from build123d import *

# Parameters (mm, degrees)
F1_DEPTH = 69.342
F4_DEPTH = 107.442
F6_DEPTH = 136.652
F7_R     = 6.789737
F7_R_2   = 6.259827
F8_DEPTH = 85.344


with BuildPart() as f1:
    # F0 (on Front) → F1 (new body)
    with BuildSketch(Plane.XZ):
        Polygon((0, 38.1), (-38.1, 38.1), (-38.1, 0), (0, 0), (38.1, 0), (38.1, 38.1), align=None)
    extrude(amount=F1_DEPTH)

    # F3 (on offset) → F4 (join)
    with BuildSketch(Plane.XZ.offset(78.994)):
        with BuildLine():
            Line((16.352327, 39.380998), (-16.352311, 39.378844))
            ThreePointArc((-16.352311, 39.378844), (0.001077, 23.146536), (16.352327, 39.380998))
        make_face()
    extrude(amount=-F4_DEPTH)

    # F5 (on offset) → F6 (cut)
    with BuildSketch(Plane.XZ.offset(78.994)):
        with BuildLine():
            Line((0, 39.475866), (-7.966925, 39.475866))
            ThreePointArc((-7.966925, 39.475866), (-0.026347, 31.508984), (7.966751, 39.423171))
            Line((7.966751, 39.423171), (0, 39.475866))
        make_face()
    extrude(amount=-F6_DEPTH, mode=Mode.SUBTRACT)

    # F7 (on Top) → F8 (cut)
    with BuildSketch(Plane.XY):
        with Locations((-27.498437, -37.382606)):
            Circle(F7_R)
        with Locations((27.498439, -37.382606)):
            Circle(F7_R_2)
    extrude(amount=F8_DEPTH, mode=Mode.SUBTRACT)


solid = f1.part
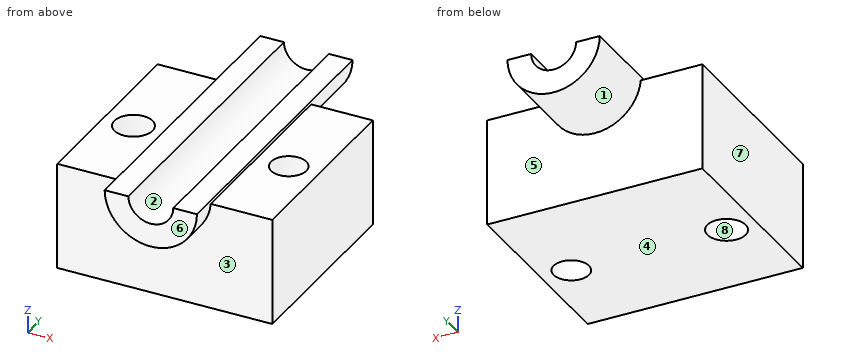
Input: part model. Units: mm. Frame: model coordinates. Face numbers are marked on the shaded views. A direction names the side the tool comes from. Coordinates: 2 decimals unless noted, no trailing zeros. Order: outer loops, then holes, each group sorted by start corner. A loop starts at its lowest first (then second) coordinate and runs counter-clockwise, first axis right, second up. Notation, with made-up numbers: M 38.25,37 L 57.25,37 A16 ccw 57.25,57 Z; hole C 59,-25.75 d2. An arc over 180 degrees is marked long. Answer in a Markdown table with one row per item.
(1) Contact query for flat-ended pins moving along their axis: pin 1 Ø19 at (x, z) = (-4.5, 14.5) entering from +Y; pin 2 Ø17.5 at (x, y) = (-25.5, -25) entering from +Z; pin 3 Ø1.5 at (x, z) = (27, 30) entering from -Y; pin 4 Ø2 at (x, z) = (-22, 19) entering from +Y. Output: stop coordinate, or through.
Numbers:
| item | result |
|---|---|
| pin 1 | stops at y = 28.45 |
| pin 2 | stops at z = 38.1 |
| pin 3 | stops at y = -69.34 |
| pin 4 | stops at y = 0 |
(2) Draft query along Y for the marked faces 6, 7 and 8. Return one class per face: pulls with the +Y half, pulls with the -Y half, needs draft (parallel to the pull), parting line crosses it, or undercut.
Numbers:
| item | result |
|---|---|
| face 6 | pulls with the -Y half |
| face 7 | needs draft |
| face 8 | undercut |
(3) Access query for the marked faces 1, 2, 3, 4 and 5. Directions: +Z, -Z, +X, -X, +Y, -Y. A direction counts if a zero-diameter tool reaches every point of the face in a straight line with its end or side. Return the directions, or none.
Numbers:
| item | result |
|---|---|
| face 1 | none |
| face 2 | +Z, +Y, -Y |
| face 3 | -Z, -Y |
| face 4 | -Z, +X, -X, +Y, -Y |
| face 5 | -Z, +Y |
(4) Section query C-C, the plane x = 0. Output: boundary loops of the cut face in (y, z), plus the area to 3 significant figures.
Numbers:
| item | result |
|---|---|
| outline | M -78.99,23.15 L -69.34,23.15 L -69.34,0 L 0,0 L 0,23.15 L 28.45,23.15 L 28.45,31.51 L -78.99,31.51 Z |
| area | 2,500 mm^2 |
(5) Section query A-A, the plane x = -31. Output: boundary loops of the cut face in (y, z), plus the area to 3 significant figures.
Numbers:
| item | result |
|---|---|
| outline | M -69.34,0 L -43.2,0 L -43.2,38.1 L -69.34,38.1 Z; M -31.57,0 L 0,0 L 0,38.1 L -31.57,38.1 Z |
| area | 2,200 mm^2 |
(6) Section query D-D, the plane x = 23. Output: boundary loops of the cut face in (y, z), plus the area to 3 significant figures.
Numbers:
| item | result |
|---|---|
| outline | M -69.34,0 L -41.74,0 L -41.74,38.1 L -69.34,38.1 Z; M -33.03,0 L 0,0 L 0,38.1 L -33.03,38.1 Z |
| area | 2,310 mm^2 |
(7) Section query B-B, the plane y = -60.5. Output: boundary loops of the cut face in (x, z).
Numbers:
| item | result |
|---|---|
| outline | M -38.1,0 L 38.1,0 L 38.1,38.1 L 16.29,38.1 A16.35 ccw 16.35,39.38 L 7.97,39.38 A7.97 cw -7.97,39.38 L -16.35,39.38 A16.35 ccw -16.29,38.1 L -38.1,38.1 Z |
(8) Material intervals for line 1 (X direction, y = -41, z = 10.5); line 2 (Y direction, x = -26, z = 5.5); line 3 (Y direction, x = 30, z = 37), sorted ascending. Write a range as [from, to].
Numbers:
| item | result |
|---|---|
| line 1 | x = [-38.1, -33.24], [-21.75, 22.39], [32.61, 38.1] |
| line 2 | y = [-69.34, -44], [-30.76, 0] |
| line 3 | y = [-69.34, -43.12], [-31.64, 0] |
